from build123d import *

# Parameters (mm, degrees)
MODEL_R             = 1.5
EXTRUDE_1_DEPTH     = 3
SKETCH_1_R          = 1.5
CUT_EXTRUDE_1_DEPTH = 10


with BuildPart() as part:
    # Model → 凸台-拉伸1 (new body)
    with BuildSketch(Plane.XY):
        with BuildLine():
            ThreePointArc((2779.510343176, 1861.218710153), (2781.63166352, 1860.340030496), (2782.510343176, 1858.218710153))
            Line((2782.510343176, 1858.218710153), (2782.510343176, 1843.218710153))
            ThreePointArc((2782.510343176, 1843.218710153), (2781.63166352, 1841.097389809), (2779.510343176, 1840.218710153))
            Line((2779.510343176, 1840.218710153), (2770.510343176, 1840.218710153))
            ThreePointArc((2770.510343176, 1840.218710153), (2768.389022832, 1839.340030496), (2767.510343176, 1837.218710153))
            Line((2767.510343176, 1837.218710153), (2767.510343176, 1744.718710153))
            Line((2767.510343176, 1744.718710153), (2767.510343176, 1730.718710153))
            Line((2767.510343176, 1730.718710153), (2787.510343176, 1730.718710153))
            Line((2787.510343176, 1730.718710153), (2792.510343176, 1730.718710153))
            Line((2792.510343176, 1730.718710153), (2812.510343176, 1730.718710153))
            Line((2812.510343176, 1730.718710153), (2812.510343176, 1732.218710153))
            Line((2812.510343176, 1732.218710153), (2812.510343176, 1737.218710153))
            Line((2812.510343176, 1737.218710153), (2812.510343176, 1744.718710153))
            Line((2812.510343176, 1744.718710153), (2812.510343176, 1970.718710153))
            Line((2812.510343176, 1970.718710153), (2767.510343176, 1970.718710153))
            Line((2767.510343176, 1970.718710153), (2767.510343176, 1864.218710153))
            ThreePointArc((2767.510343176, 1864.218710153), (2768.389022832, 1862.097389809), (2770.510343176, 1861.218710153))
            Line((2770.510343176, 1861.218710153), (2779.510343176, 1861.218710153))
        make_face()
        with Locations((2771.510343176, 1741.218710153)):
            Circle(MODEL_R, mode=Mode.SUBTRACT)
        with Locations((2783.510343176, 1741.218710153)):
            Circle(MODEL_R, mode=Mode.SUBTRACT)
        with Locations((2770.510343176, 1827.618710153)):
            Circle(MODEL_R, mode=Mode.SUBTRACT)
        with Locations((2784.510343176, 1827.618710153)):
            Circle(MODEL_R, mode=Mode.SUBTRACT)
        with Locations((2796.510343176, 1741.218710153)):
            Circle(MODEL_R, mode=Mode.SUBTRACT)
        with Locations((2808.510343176, 1741.218710153)):
            Circle(MODEL_R, mode=Mode.SUBTRACT)
        with Locations((2770.510343176, 1873.818710153)):
            Circle(MODEL_R, mode=Mode.SUBTRACT)
        with Locations((2784.510343176, 1873.818710153)):
            Circle(MODEL_R, mode=Mode.SUBTRACT)
        with Locations((2771.510343176, 1960.218710153)):
            Circle(MODEL_R, mode=Mode.SUBTRACT)
        with Locations((2783.510343176, 1960.218710153)):
            Circle(MODEL_R, mode=Mode.SUBTRACT)
        with Locations((2796.510343176, 1960.218710153)):
            Circle(MODEL_R, mode=Mode.SUBTRACT)
        with Locations((2808.510343176, 1960.218710153)):
            Circle(MODEL_R, mode=Mode.SUBTRACT)
    extrude(amount=EXTRUDE_1_DEPTH)

    # 草图1 → 切除-拉伸1 (cut)
    with BuildSketch(Plane.XY.offset(3)):
        with Locations((2770.510343176, 1794.618710153)):
            Circle(SKETCH_1_R)
        with Locations((2784.510343176, 1794.618710153)):
            Circle(SKETCH_1_R)
    extrude(amount=-CUT_EXTRUDE_1_DEPTH, mode=Mode.SUBTRACT)


solid = part.part
Source: CAD feature listing. Evaluate the final solid. Frame: model axes, mm. Round coordinates to 2 decimals unless told otherwise and drop trailing zeros. Return JSON: item names as keys, results as strings. Group by question number.
1. Section query A-A on z = 1.75. State how many separate pieces and enclosed holes the cut face has, and give its area (3 significant figures).
2. Pin query (flat end, axial travel): pin 1 (2.5 mm diameter, centred on x = 2770.51, y = 1827.62, fed in from +Z). Return the tip coordinate at first contact, or that it passes through.
3. Material intervals for line 1 along X through (y, z) = (1795, 2.8); line 2 along Y through (x, z) = (2778.5, 2.1); line 3 along Y through (x, z) = (2807.5, 2.3), sorted ascending. Write a range as from..to.
Checks:
{
 "1": {"separate pieces": "1", "enclosed holes": "14", "area": "10,400 mm²"},
 "2": {"pin 1": "passes through"},
 "3": {"line 1": "x = 2767.51..2769.06, 2771.96..2783.06, 2785.96..2812.51", "line 2": "y = 1730.72..1840.22, 1861.22..1970.72", "line 3": "y = 1730.72..1740.11, 1742.33..1959.11, 1961.33..1970.72"}
}
